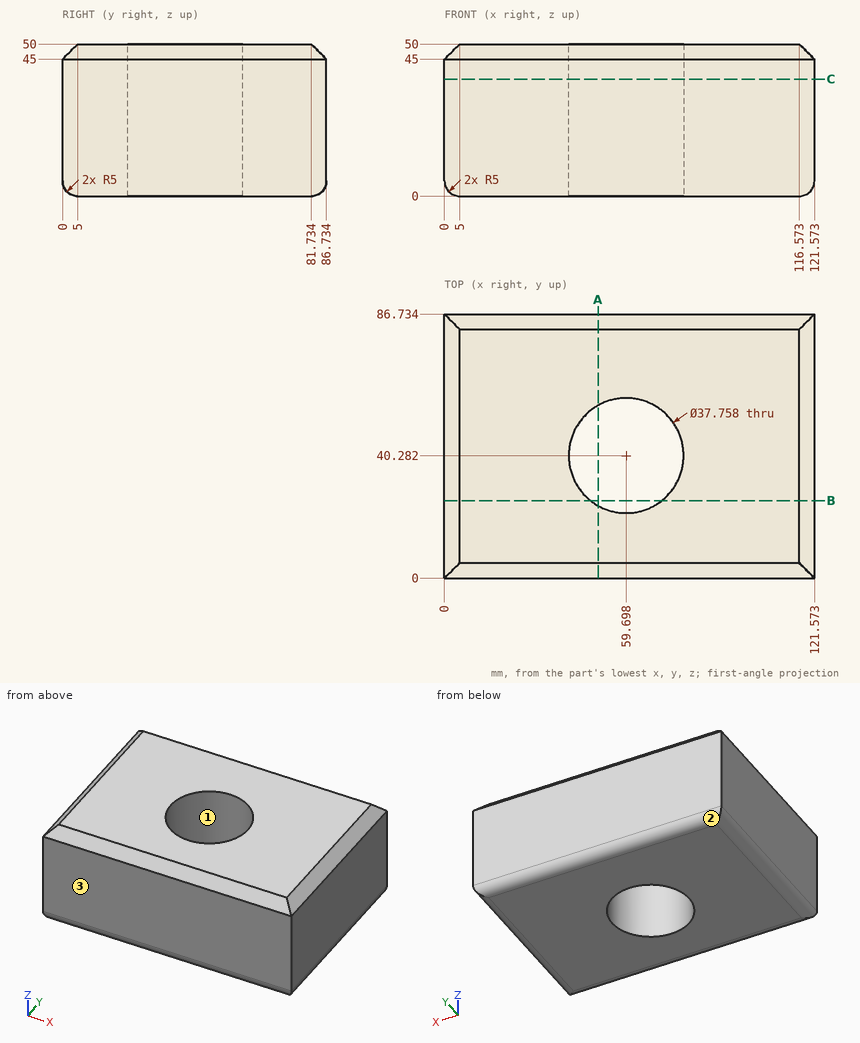
Print and shaded views of the part. All mm, measured from the part's lowest x, y and z. Give positions to 0.01 mm unless a question says otherwise; leave off trailing zeros. Loops run counter-clockwise (first coordinate to the right, second up) from the corner with the lowest first, then second, coordinate; pieces in that order, holes last. Notation, with made-up numbers: (-9, 27) -> (6, 27) arc R27 ccw to (6, 62) -> close; hole circle Ø11 at (71, -14.75). An arc over 180 degrees is marked (long way). One line per question, with ' | ' between items. Start each with the question number.
1) Probe L1, parallel to X at y = 38, z = 23.5; L2, parallel to X at y = 51, z = 16.5 (1 decimal); L3, parallel to Y at x = 74.5, z = 26 (1 decimal). List the from-to ranges inside material, lowest first.
2) Cut at C-C (z = 38.5). Give the cut face in (x, y).
3) Two-plate mould, pull along Y, no slides. Class the marked faces 1, 2 and 3: released by +Y, released by -Y, zero draft, split by the parting line, or undercut.
4) Cut at B-B (y = 25.5). Give the cut face in (x, z) (1 decimal).
5) Cut at A-A (x = 50.5). Give the cut face in (y, z) (1 decimal).
Return value:
1) L1: 0 to 40.96, 78.44 to 121.57 | L2: 0 to 44.2, 75.2 to 121.6 | L3: 0 to 28.6, 52 to 86.7
2) outline: (0, 0) -> (121.57, 0) -> (121.57, 86.73) -> (0, 86.73) -> close; hole circle Ø37.76 at (59.7, 40.28)
3) face 1: undercut | face 2: released by +Y | face 3: released by -Y
4) outline: (0, 5) arc R5 ccw to (5, 0) -> (48, 0) -> (48, 50) -> (5, 50) -> (0, 45) -> close; (71.4, 0) -> (116.6, 0) arc R5 ccw to (121.6, 5) -> (121.6, 45) -> (116.6, 50) -> (71.4, 50) -> close
5) outline: (0, 5) arc R5 ccw to (5, 0) -> (23.8, 0) -> (23.8, 50) -> (5, 50) -> (0, 45) -> close; (56.8, 0) -> (81.7, 0) arc R5 ccw to (86.7, 5) -> (86.7, 45) -> (81.7, 50) -> (56.8, 50) -> close
